from build123d import *

# Parameters (mm, degrees)
PAD_DEPTH        = 10
FILLET_R         = 2
FILLET001_R      = 2
HOLE_D           = 6.6
HOLE_DEPTH       = 25
HOLE_CBORE_D     = 11
HOLE_CBORE_DEPTH = 6.4


with BuildPart() as part:
    # Sketch → Pad (new body)
    with BuildSketch(Plane.XY):
        with BuildLine():
            Line((-21.9, 24.9), (21.9, 24.9))
            ThreePointArc((24.9, 21.9), (24.02132, 24.02132), (21.9, 24.9))
            Line((24.9, 21.9), (24.9, -21.9))
            ThreePointArc((21.9, -24.9), (24.02132, -24.02132), (24.9, -21.9))
            Line((21.9, -24.9), (-21.9, -24.9))
            ThreePointArc((-24.9, -21.9), (-24.02132, -24.02132), (-21.9, -24.9))
            Line((-24.9, -21.9), (-24.9, 21.9))
            ThreePointArc((-21.9, 24.9), (-24.02132, 24.02132), (-24.9, 21.9))
        make_face()
        with BuildLine():
            ThreePointArc((-9.4, 13), (-12.5, 16.1), (-15.6, 13))
            Line((-15.6, 13), (-15.6, -13))
            ThreePointArc((-15.6, -13), (-12.5, -16.1), (-9.4, -13))
            Line((-9.4, -13), (-9.4, 13))
        make_face(mode=Mode.SUBTRACT)
        with BuildLine():
            ThreePointArc((15.6, 13), (12.5, 16.1), (9.4, 13))
            Line((9.4, 13), (9.4, -13))
            ThreePointArc((9.4, -13), (12.5, -16.1), (15.6, -13))
            Line((15.6, -13), (15.6, 13))
        make_face(mode=Mode.SUBTRACT)
    extrude(amount=PAD_DEPTH)

    # Fillet
    fillet_edges = [part.edges().sort_by_distance(p)[0] for p in [
        (0, -24.9, 10),
    ]]
    fillet(fillet_edges, radius=FILLET_R)

    # Fillet001
    fillet001_edges = [part.edges().sort_by_distance(p)[0] for p in [
        (0, -24.9, 0),
    ]]
    fillet(fillet001_edges, radius=FILLET001_R)

    # Hole
    with Locations(Plane.XY.offset(10)):
        with Locations((0, 0), (0, 12.5), (0, -12.5)):
            CounterBoreHole(HOLE_D / 2, HOLE_CBORE_D / 2, HOLE_CBORE_DEPTH, depth=HOLE_DEPTH)


solid = part.part
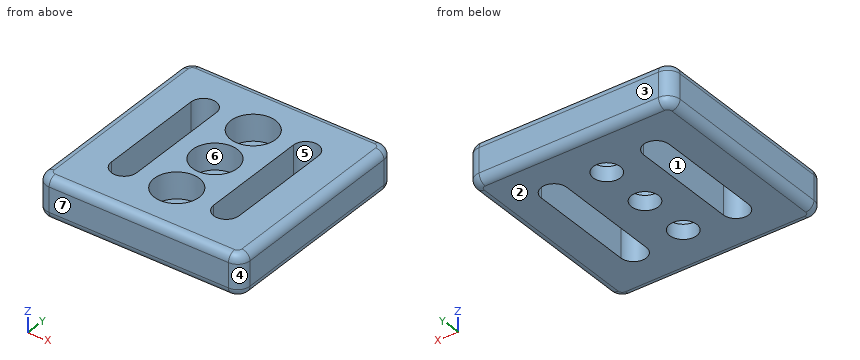
Could you check a few things on this model? Use its own coordinates, in mm. Face numbers are marked on the shaded views. A direction names the side the tool comes from. Give positions to 0.01 mm unless a question says otherwise; leave off trailing zeros. Loops run counter-clockwise (first coordinate to the right, second up) from the corner with the lowest first, then second, coordinate; pieces in that order, holes last. Notation, with made-up numbers: (67.25, 65.5) -> (119.25, 65.5) arc R18 ccw to (119.25, 72.5) -> close; hole circle Ø4 at (-19.75, 25.5). An arc over 180 degrees is marked (long way). Return JSON: item names as keys, results as strings.
Item 1: If we section it at C-C on x = 0: Count the separate pieces of the cut face and the enclosed holes in it, plus the area to 3 significant figures.
Geometry results:
{"separate pieces": "4", "enclosed holes": "0", "area": "212 mm²"}
Item 2: I need wall thicknesses on L1, parallel to Y at x = 0, z = 5.25; L2, parallel to Y at x = 0, z = 2.05; L3, parallel to X at y = -5, z = 2. Which ranges of each line are inside material? Lowest first, please. Write a range as from..to.
Geometry results:
{"L1": "y = -24.9..-18, -7..-5.5, 5.5..7, 18..24.9", "L2": "y = -24.9..-15.8, -9.2..-3.3, 3.3..9.2, 15.8..24.9", "L3": "x = -24.9..-15.6, -9.4..9.4, 15.6..24.9"}
Item 3: We'd pull the mould along Y, two halves only. Please class the marked faces 1, 2, 3 and 4: +Y half, -Y half, draft (parallel to the pull), parting line (faces both ways), or undercut.
Geometry results:
{"face 1": "undercut", "face 2": "draft", "face 3": "+Y half", "face 4": "-Y half"}
Item 4: If we section it at A-A on y = 0: List the corners of the cut face in (x, z) for me, plus the area to 3 significant figures.
Geometry results:
{"outline": "(-24.9, 2) arc R2 ccw to (-22.9, 0) -> (-15.6, 0) -> (-15.6, 10) -> (-22.9, 10) arc R2 ccw to (-24.9, 8) -> close; (-9.4, 0) -> (-3.3, 0) -> (-3.3, 3.6) -> (-5.5, 3.6) -> (-5.5, 10) -> (-9.4, 10) -> close; (3.3, 0) -> (9.4, 0) -> (9.4, 10) -> (5.5, 10) -> (5.5, 3.6) -> (3.3, 3.6) -> close; (15.6, 0) -> (22.9, 0) arc R2 ccw to (24.9, 2) -> (24.9, 8) arc R2 ccw to (22.9, 10) -> (15.6, 10) -> close", "area": "276 mm²"}
Item 5: Which directions (+Z, -Z, +X, -X, +Y, -Y) give clear straight access to the entire face, cutting with the end or side of a thin tool? Please do the marked faces 5, 6 and 7.
Geometry results:
{"face 5": "+Z, -Z", "face 6": "+Z", "face 7": "+Z, -Z, +X, -X, -Y"}
Item 6: If we section it at D-D on y = -10: List the corners of the cut face in (x, z) for me.
Geometry results:
{"outline": "(-24.9, 2) arc R2 ccw to (-22.9, 0) -> (-15.6, 0) -> (-15.6, 10) -> (-22.9, 10) arc R2 ccw to (-24.9, 8) -> close; (-9.4, 0) -> (-2.15, 0) -> (-2.15, 3.6) -> (-4.9, 3.6) -> (-4.9, 10) -> (-9.4, 10) -> close; (2.15, 0) -> (9.4, 0) -> (9.4, 10) -> (4.9, 10) -> (4.9, 3.6) -> (2.15, 3.6) -> close; (15.6, 0) -> (22.9, 0) arc R2 ccw to (24.9, 2) -> (24.9, 8) arc R2 ccw to (22.9, 10) -> (15.6, 10) -> close"}
Item 7: I'm going to push flat-ended pins straight in: pin 1 (6 mm diameter, centred on x = 0, y = -12.5, fed in from -Z); pin 2 (3.5 mm diameter, centred on x = -2.5, y = -15, fed in from +Z). Where does each tip first touch, or does it pass through?
Geometry results:
{"pin 1": "passes through", "pin 2": "stops at z = 3.6"}
Item 8: If we section it at B-B on x = 12.5: List the corners of the cut face in (y, z) for me, plus the area to 3 significant figures.
Geometry results:
{"outline": "(-24.9, 2) arc R2 ccw to (-22.9, 0) -> (-16.1, 0) -> (-16.1, 10) -> (-22.9, 10) arc R2 ccw to (-24.9, 8) -> close; (16.1, 0) -> (22.9, 0) arc R2 ccw to (24.9, 2) -> (24.9, 8) arc R2 ccw to (22.9, 10) -> (16.1, 10) -> close", "area": "173 mm²"}
